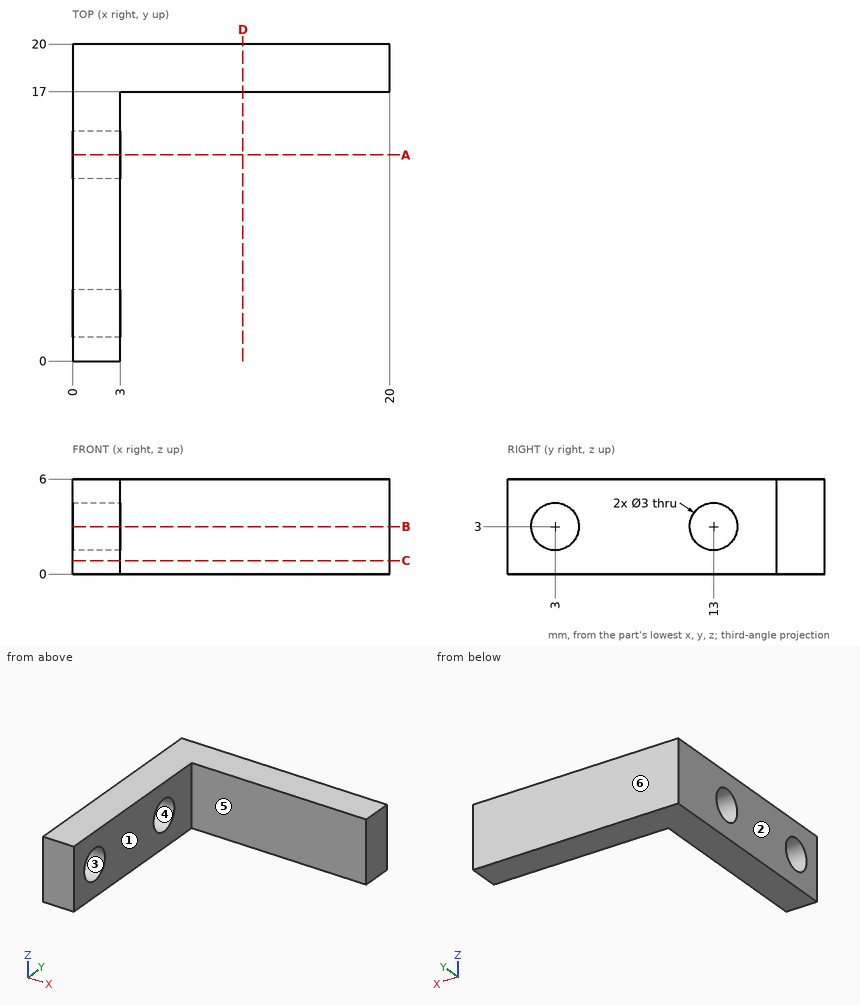
Design review of the part shown in the three views and the two pictorial views. Dimensions are in mm from the part's minimum x, y and z. A direction names the side the tool comes from. Give positions to 0.01 mm unless a question says otherwise; leave off trailing zeros. Loops run counter-clockwise (first coordinate to the right, second up) from the corner with the lowest first, then second, coordinate; pieces in that order, holes last. Notation, with made-up numbers: (25, -10.5) -> (62, -10.5) arc R20 cw to (62, 25.5) -> close; hole circle Ø8 at (63.25, 59). An arc over 180 degrees is marked (long way). One line per item, written item: value.
Q1. We need section A-A on y = 13. Give the boundary of the cut face in (x, z).
Numbers:
outline: (0, 0) -> (3, 0) -> (3, 1.5) -> (0, 1.5) -> close; (0, 4.5) -> (3, 4.5) -> (3, 6) -> (0, 6) -> close
Q2. We need section C-C on z = 0.85. Give the boundary of the cut face in (x, y), and give its area (3 significant figures).
Numbers:
outline: (0, 0) -> (3, 0) -> (3, 17) -> (20, 17) -> (20, 20) -> (0, 20) -> close
area: 111 mm^2
Q3. We need section D-D on x = 10.75. Give the boundary of the cut face in (y, z).
Numbers:
outline: (17, 0) -> (20, 0) -> (20, 6) -> (17, 6) -> close
Q4. Draft analysis for pull direction Y (two halves, no side actions). For the marked faces 3, 4, 5 and 6, state which applies: pulls with the +Y half, pulls with the -Y half, needs draft (parallel to the pull), parting line crosses it, or undercut.
Numbers:
face 3: undercut
face 4: undercut
face 5: pulls with the -Y half
face 6: pulls with the +Y half
Q5. For pin 1 Ø3 at (y, z) = (9, 4) entering from +X; pin 2 Ø1 at (x, y) = (5.5, 15) entering from +Z; pin 3 Ø1.8 at (x, z) = (14.5, 4) entering from -Y, all flat-tipped, find the tip position at first contact; note any pin that passes through.
Numbers:
pin 1: stops at x = 3
pin 2: passes through
pin 3: stops at y = 17
Q6. Machinability: for the marked faces 1 and 2, which of the approach directions +Z, -Z, +X, -X, +Y, -Y give a long, thin tool a straight path to every point of the face, cutting with its end or side? Answer none if there is none.
Numbers:
face 1: +Z, -Z, +X, -Y
face 2: +Z, -Z, -X, +Y, -Y
Q7. For L1, parallel to Y at x = 2.1, z = 3; L2, parallel to X at y = 5.75, z = 1.8; L3, parallel to Y at x = 15, z = 5.5, list the stretches that pass through material, from the lowest coordinate up.
Numbers:
L1: y = 0 to 1.5, 4.5 to 11.5, 14.5 to 20
L2: x = 0 to 3
L3: y = 17 to 20
Q8. We need section B-B on z = 3. Give the boundary of the cut face in (x, y).
Numbers:
outline: (0, 0) -> (3, 0) -> (3, 1.5) -> (0, 1.5) -> close; (0, 4.5) -> (3, 4.5) -> (3, 11.5) -> (0, 11.5) -> close; (0, 14.5) -> (3, 14.5) -> (3, 17) -> (20, 17) -> (20, 20) -> (0, 20) -> close
